Geometry check sheet. Reference: the model listing, model coordinates, mm. A direction names the side the tool comes from. Coordinates: 2 decimals unless noted, no trailing zeros. Write each loop counter-clockwise with the first axis right and the second up, starting at its lowest first coordinate (ties: lowest second). Pieces come first, ordered by that corner, then holes. Notation, with made-up numbers: M 33,10 L 83,10 A22 ccw 83,44 Z; hole C -36.5,-20.75 d1. An arc over 180 degrees is marked long. Put each result on its own line as item: value. Start each with the question number.
1) Gauge pin test, flat ends, axial feed: pin 1 (2.5 mm diameter, centred on x = 0, z = 5.5, fed in from +Y); pin 2 (1.5 mm diameter, centred on y = 9.5, z = 3, fed in from -X); pin 3 (1 mm diameter, centred on x = 0, y = 1, fed in from -Z); pin 4 (3.5 mm diameter, centred on x = -0.5, z = 2.5, fed in from +Y). Record the tip position at first contact, or that the pin passes through.
2) Cross-section at A-A on y = 13.75. Record the cut outline in (x, z), plus the area to 3 significant figures.
3) Scan lines: line 1 along X through (y, z) = (1, 1.75); line 2 along Y through (x, z) = (-0.25, 5.5); line 3 along X through (y, z) = (17.5, 1.5). Record each from-to range of solid material in increasing order.
4) Mould release check, pull along Y, two halves, no side actions. Record for faces 4 (the cylindrical face through (2.98, -2.95, 4.93)), 5 (the flat face through (-3.2, 14, 5)), 6 (the flat face through (0, 2.05, 5)): released by +Y, released by -Y, zero draft, split by the parting line, or undercut.
5) Cross-section at D-D on x = -2.5. Record the cut outline in (y, z), plus the area to 3 significant figures.
6) Cross-section at C-C on z = 6.25. Record the cut outline in (x, y).
7) Set-up check for faces 1 (the flat face through (3.55, 3, 5)), 2 (the flat face through (-1.7, 14, 5)), 3 (the flat face through (-2.05, 0, 5)): record each of +Z, -Z, +X, -X, +Y, -Y from which the full face is reachable in a straight line by a thin tool's end or side.
8) Cross-section at B-B on x = 1.25. Record the cut outline in (y, z).
Autodesk Inventor part; units mm, degrees
ref_plane "YZ Plane" through (0, 0, 0) normal (1, 0, 0) x (0, 1, 0)
ref_plane "XZ Plane" through (0, 0, 0) normal (0, 1, 0) x (-1, 0, 0)
ref_plane "XY Plane" through (0, 0, 0) normal (0, 0, 1) x (1, 0, 0)
sketch "Sketch1" plane through (0, 0, 0) normal (0, 0, 1) x (1, 0, 0)
  line L0 (-2.05, 2.05) -> (2.05, 2.05)
  line L1 (2.05, 2.05) -> (2.05, -2.05)
  line L2 (2.05, -2.05) -> (-2.05, -2.05)
  line L3 (-2.05, -2.05) -> (-2.05, 2.05)
  line L4 (0, 2.05) -> (0, -2.05) construction
  line L5 (0, 7.5) -> (-15.55, 7.5)
  line L6 (-15.55, 7.5) -> (-15.55, 6)
  line L7 (-15.55, 6) -> (-3.55, 6)
  line L8 (-3.55, 6) -> (-3.55, -6)
  line L9 (-3.55, -6) -> (-15.55, -6)
  line L10 (-15.55, -6) -> (-15.55, -7.5)
  line L11 (-15.55, -7.5) -> (-0.55, -7.5)
  line L12 (-2.05, 0) -> (2.05, 0) construction
  line L13 (0, 7.5) -> (15.55, 7.5)
  line L14 (15.55, 7.5) -> (15.55, 6)
  line L15 (15.55, 6) -> (3.55, 6)
  line L16 (3.55, 6) -> (3.55, -6)
  line L17 (3.55, -6) -> (15.55, -6)
  line L18 (15.55, -6) -> (15.55, -7.5)
  line L19 (15.55, -7.5) -> (-0.55, -7.5)
  line L20 (-2.05, 2.05) -> (2.05, -2.05) construction
  line L21 (2.05, 2.05) -> (-2.05, -2.05) construction
  line L22 (0, 7.5) -> (0, 2.05) construction
  line L23 (-3.55, 6) -> (-3.55, 7.5)
  line L24 (-3.55, -6) -> (-3.55, -7.5)
  line L25 (3.55, 6) -> (3.55, 7.5)
  line L26 (3.55, -6) -> (3.55, -7.5)
  point P0 (0, 0)
  point P1 (0, 0)
  point P2 (0, 0)
  dimension "d3" = 4.1
  dimension "d4" = 4.1
  dimension "d5" = 12
  dimension "d6" = 1.5
  dimension "d7" = 1.5
  dimension "d8" = 5.45
  dimension "d9" = 5.45
  dimension "d10" = 1.5
  dimension "d11" = 12
  dimension "d37" = 15
extrude "Extrusion1" add sketch "Sketch1" along normal blind 10 contours L13 L25 L16 L26 L19 L11 L24 L8 L23 L5
sketch "Sketch5" plane through (0, 0, 10) normal (0, 0, 1) x (1, 0, 0)
  line L0 (1.7, 19.5) -> (3.2, 19.5)
  line L1 (3.2, 19.5) -> (3.2, 7.5)
  line L2 (3.2, 7.5) -> (1.7, 7.5)
  line L3 (1.7, 7.5) -> (1.7, 19.5)
  line L4 (3.55, 7.5) -> (-3.55, 7.5)
  line L5 (3.55, -7.5) -> (3.55, 7.5)
  line L6 (0, 0) -> (0, 23.4065) construction
  point P0 (15.55, 7.5)
  point P1 (-15.55, 7.5)
  point P2 (3.55, -6)
  point P3 (3.55, 6)
  dimension "d41" = 1.5
  dimension "d42" = 12
  dimension "d47" = 1.7
extrude "Extrusion5" add sketch "Sketch5" against normal up to surface (10 mm away)
mirror "Mirror1" about plane through (0, 0, 0) normal (1, 0, 0) of "Extrusion5"
sketch "Sketch8" plane through (0, 0, 10) normal (0, 0, 1) x (1, 0, 0)
  line L0 (-3.55, -3.55) -> (3.55, -3.55)
  line L1 (3.55, -3.55) -> (3.55, -7.5)
  line L2 (3.55, -7.5) -> (-3.55, -7.5)
  line L3 (-3.55, -7.5) -> (-3.55, -3.55)
  line L4 (2.05, -2.05) -> (-2.05, -2.05)
  line L5 (3.55, -7.5) -> (3.55, 7.5)
  line L6 (-3.55, 7.5) -> (-3.55, -7.5)
  line L7 (-3.55, -7.5) -> (3.55, -7.5)
  point P0 (0, 0)
  point P1 (3.55, 5)
  point P2 (-3.55, 5)
  dimension "d57" = 1.5
extrude "Extrusion8" cut sketch "Sketch8" against normal blind 10
fillet "Fillet4" radius 2 4 edges at (-2.45, 19.5, 10) (-2.45, 19.5, 0) (2.45, 19.5, 0) (2.45, 19.5, 10)
fillet "Fillet5" radius 2 2 edges at (3.55, -3.55, 5) (-3.55, -3.55, 5)
fillet "Fillet6" radius 2 2 edges at (-3.2, 7.5, 5) (3.2, 7.5, 5)
equation "\"d7\" = d6"
equation "\"d8\" = d9"
properties part number "fuselage_tail_interface_airfoiled_v2" material "ABS Plastic"
Answer key:
1. pin 1: stops at y = 7.5
1. pin 2: stops at x = -3.2
1. pin 3: passes through
1. pin 4: stops at y = 19.5
2. outline: M -3.2,0 L -1.7,0 L -1.7,10 L -3.2,10 Z; M 1.7,0 L 3.2,0 L 3.2,10 L 1.7,10 Z
2. area: 30.0 mm²
3. line 1: x = -3.55 to -2.05, 2.05 to 3.55
3. line 2: y = -3.55 to -2.05, 2.05 to 7.5
3. line 3: x = -3.2 to -1.7, 1.7 to 3.2
4. face 4: released by -Y
4. face 5: zero draft
4. face 6: undercut
5. outline: M -3.31,0 L 17.5,0 A2 ccw 19.5,2 L 19.5,8 A2 ccw 17.5,10 L -3.31,10 Z
5. area: 226 mm²
6. outline: M -3.55,-1.55 A2 ccw -1.55,-3.55 L 1.55,-3.55 A2 ccw 3.55,-1.55 L 3.55,7.5 A2 cw 3.2,8.63 L 3.2,19.5 L 1.7,19.5 L 1.7,7.5 L -1.7,7.5 L -1.7,19.5 L -3.2,19.5 L -3.2,8.63 A2 cw -3.55,7.5 Z; hole M -2.05,-2.05 L 2.05,-2.05 L 2.05,2.05 L -2.05,2.05 Z
7. face 1: +Z, -Z, +X, +Y, -Y
7. face 2: +Z, -Z, +Y
7. face 3: +Z, -Z
8. outline: M -3.55,0 L -2.05,0 L -2.05,10 L -3.55,10 Z; M 2.05,0 L 7.5,0 L 7.5,10 L 2.05,10 Z
